from build123d import *

# Parameters (mm, degrees)
F1_DEPTH = 34.036
F3_DEPTH = 25.4
F4_DEPTH = 25.4


with BuildPart() as f1:
    # F0 (on Top) → F1 (new body)
    with BuildSketch(Plane.XY):
        Polygon((0, 61.9426332414), (-11.7109799758, 23.0268388987), (-48.476384759, 17.6629981817), (-12.558279559, 5.6331055239), (-24.2008212954, -29.1284713894), (0, -8.3885807544), (34.6354208887, -31.8980328739), (12.4329142272, 4.1770320386), (54.0130585432, 15.7661139965), (12.4329142272, 23.1984425336), align=None)
    extrude(amount=F1_DEPTH)

    # F2 (on face) → F3 (join)
    with BuildSketch(Plane.XY.offset(34.036)):
        Polygon((-0.6540262179, 35.5291943997), (-6.1076348647, 17.4067560583), (-17.9816167802, 16.7758520693), (-4.5490903707, 8.2113984972), (-8.1022512168, -3.595818067), (0, 4.1770320386), (14.4822600718, -4.6202587845), (6.5849781968, 8.2113984972), (24.167701602, 16.7758520693), (6.5849781968, 19.013568759), align=None)
    extrude(amount=F3_DEPTH)

    # F4 (add): faces of the model
    f4_faces = [f1.faces().sort_by_distance(p)[0] for p in [
        (2.0638744173, 13.7880141108, 59.436),
        (2.0271315912, 10.6742348057, 0),
    ]]
    extrude(f4_faces, amount=F4_DEPTH, dir=(0, 0, 1))


solid = f1.part
Source: CAD feature listing. Evaluate the final solid. Frame: model axes, mm. A direction names the side the tool comes from. Give positions to 0.01 mm unless a question says otherwise; leave off trailing zeros. Order: outer loops, then holes, each group sorted by start corner. A loop starts at its lowest first (then second) coordinate and runs counter-clockwise, first axis right, second up. Notation, with made-up numbers: (24, 83) -> (57, 83) arc R25 ccw to (57, 109) -> close; hole circle Ø5 at (68.5, 70). An arc over 180 degrees is marked (long way). Use a Markdown table: item, result.
1) Contact query for flat-ended pins moving along their axis: P1, Ø8, axis at y = 45.5, z = 26, coming from the -X side; P2, Ø8, axis at x = 35, y = -21.5, coming from the +Z side; P3, Ø3, axis at x = 11.5, z = 68, coming from the -Y side; P4, Ø1, axis at x = 16, z = 72.5, coming from the -Y side. Output: stop coordinate, or through.
Answer list:
| item | result |
|---|---|
| P1 | x = -6.15 |
| P2 | through |
| P3 | y = -3.72 |
| P4 | y = 12.55 |
2) Ray query, line 1 along Z through (x, y) = (-2, -1.5); line 2 along X through (y, z) = (-27, 33); line 3 along X through (y, z) = (10.5, 67). Return the intervals inside material, ascending. Write a range as [from, to].
Answer list:
| item | result |
|---|---|
| line 1 | [0, 34.04] |
| line 2 | [-23.49, -21.72], [27.42, 31.62] |
| line 3 | [-8.14, 11.28] |
3) Section query C-C, the plane y = 12. Return the cut outline in (x, z), then the cut area to 3 significant figures.
Answer list:
| item | result |
|---|---|
| outline | (-31.57, 0) -> (40.5, 0) -> (40.5, 34.04) -> (14.36, 34.04) -> (14.36, 84.84) -> (-10.49, 84.84) -> (-10.49, 34.04) -> (-31.57, 34.04) -> close |
| area | 3,720 mm² |
4) Reachability of faces 4 (the flat face through (-12.27, -18.904, 16.78)), 5 (the flat face through (23.69, -14.11, 16.78)), 6 (the flat face through (-18.298, -11.504, 16.78)) from +Z, -Z, +X, -X, +Y, -Y: full face, straight path, thin tool, end or side. Return the list, or none.
Answer list:
| item | result |
|---|---|
| face 4 | +Z, -Z, -Y |
| face 5 | +Z, -Z, +X |
| face 6 | +Z, -Z, -X |
5) Section query A-A, the plane z = 23.5. Return the cut outline in (x, y), then the cut area to 3 significant figures.
Answer list:
| item | result |
|---|---|
| outline | (-48.48, 17.66) -> (-12.56, 5.63) -> (-24.2, -29.13) -> (0, -8.39) -> (34.64, -31.9) -> (12.43, 4.18) -> (54.01, 15.77) -> (12.43, 23.2) -> (0, 61.94) -> (-11.71, 23.03) -> close |
| area | 2,460 mm² |
6) Mould query, pull axis Y, two halves, no side actions, for faces 1 (the flat face through (-30.769, 11.732, 16.78)), 2 (the flat face through (3.016, 27.156, 59.08)), 3 (the flat face through (7.14, -0.16, 59.08)). Classes: +Y half, -Y half, draft (parallel to the pull), parting line (faces both ways), or undercut.
Answer list:
| item | result |
|---|---|
| face 1 | undercut |
| face 2 | +Y half |
| face 3 | -Y half |
7) Section query B-B, the plane x = -16. Return the cut outline in (y, z), then the cut area to 3 significant figures.
Answer list:
| item | result |
|---|---|
| outline | (-22.1, 0) -> (-4.64, 0) -> (-4.64, 34.04) -> (-22.1, 34.04) -> close; (6.79, 0) -> (22.4, 0) -> (22.4, 34.04) -> (16.88, 34.04) -> (16.88, 84.84) -> (15.51, 84.84) -> (15.51, 34.04) -> (6.79, 34.04) -> close |
| area | 1,200 mm² |
8) Section query D-D, the plane y = -19. Return the cut outline in (x, z), then the cut area to 3 significant figures.
Answer list:
| item | result |
|---|---|
| outline | (-20.81, 0) -> (-12.38, 0) -> (-12.38, 34.04) -> (-20.81, 34.04) -> close; (15.63, 0) -> (26.7, 0) -> (26.7, 34.04) -> (15.63, 34.04) -> close |
| area | 663 mm² |
